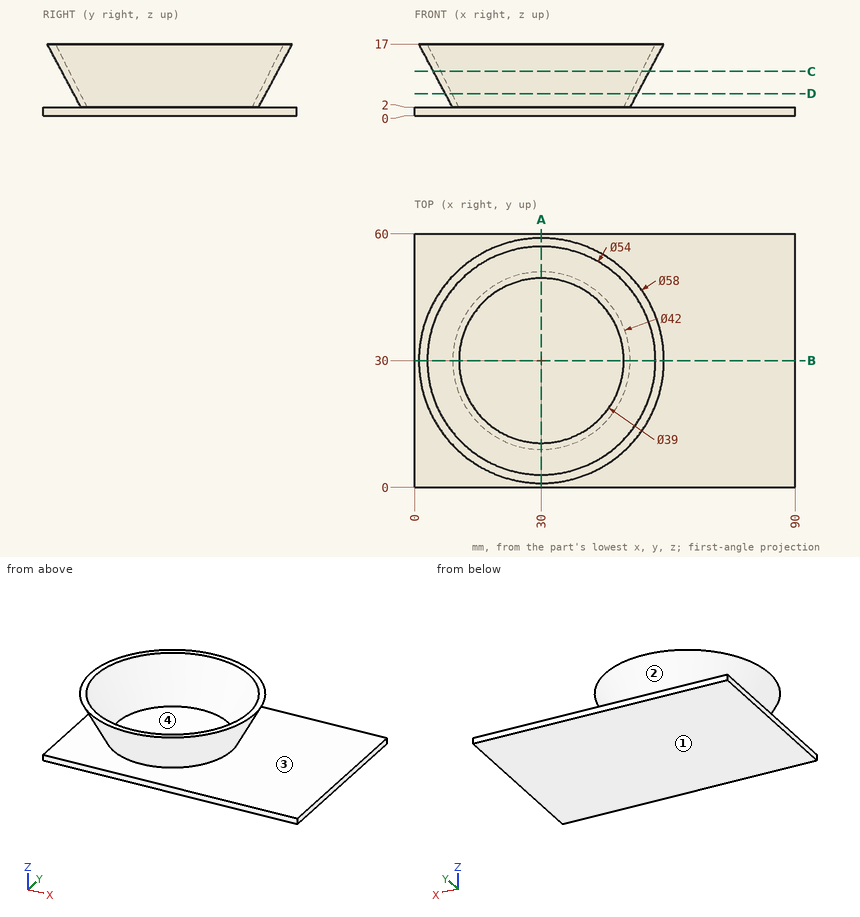
The figure shows three views and two pictorial views of one solid part (mm, origin at its lowest corner). Answer the questions. A direction names the side the tool comes from. Round coordinates to 2 decimals unless told otherwise and drop trailing zeros. Write each loop counter-clockwise with the first axis right and the second up, starting at its lowest first coordinate (ties: lowest second). Pieces come first, ordered by that corner, then holes. Notation, with made-up numbers: (-36, 64) - (4, 64) arc R25 cw to (4, 85) - close; hole circle Ø10 at (20.25, -7.75). An arc over 180 degrees is marked (long way). Use one line per item in the form item = value. Start each with the question number.
Item 1: Determine the mould class of the marked faces 3 and 4 for opening direction X: +X half, -X half, draft (parallel to the pull), parting line (faces both ways), or undercut.
Item 2: A cutting plane is placed at B-B (y = 30). Write down the section's boundary in (x, z), plus the area to 4 significant figures.
Item 3: A cutting plane is placed at D-D (z = 5.25). Write down the section's boundary in (x, y) (3 decimals), plus the area to 3 significant figures.
Item 4: A cutting plane is placed at A-A (x = 30). Write down the section's boundary in (y, z), plus the area to 4 significant figures.
Item 5: Find the intervals of material crossed by line 1 (X direction, y = 39, z = 14.75); line 2 (X direction, y = 15.5, z = 8.75); line 3 (Y direction, x = 16.5, z = 7.5), in increasing order. Write a range as [from, to].
Item 6: A cutting plane is placed at C-C (z = 10.5). Write down the section's boundary in (x, y), plus the area to 3 significant figures.
Item 7: A tool of negligible diameter and unlimited length cuts with its end or side. For the marked faces 1 and 2, from which of +Z, -Z, +X, -X, +Y, -Y can it reach the whole face along a straight path? Write none if from no direction.
Item 8: Flat-ended cylindrical pins translate along their axes: pin 1 Ø8 at (x, y) = (32.5, 52.5) entering from +Z; pin 2 Ø6 at (x, z) = (35.5, 9) entering from -Y; pin 3 Ø19.5 at (x, y) = (29, 20.5) entering from +Z. Find the tip coordinate at first contact, or state that the pin passes through.
The answers:
q1.face_3 = draft
q1.face_4 = undercut
q2.outline = (0, 0) - (90, 0) - (90, 2) - (51, 2) - (59, 17) - (57, 17) - (49.5, 2) - (10.5, 2) - (3, 17) - (1, 17) - (9, 2) - (0, 2) - close
q2.area = 232.5 mm^2
q3.outline = circle Ø45.467 at (30, 30); hole circle Ø42.25 at (30, 30)
q3.area = 222 mm^2
q4.outline = (0, 0) - (60, 0) - (60, 2) - (51, 2) - (59, 17) - (57, 17) - (49.5, 2) - (10.5, 2) - (3, 17) - (1, 17) - (9, 2) - (0, 2) - close
q4.area = 172.5 mm^2
q5.line_1 = [3.7, 5.74], [54.26, 56.3]
q5.line_2 = [10.13, 12.31], [47.69, 49.87]
q5.line_3 = [10.24, 12.31], [47.69, 49.76]
q6.outline = circle Ø51.07 at (30, 30); hole circle Ø47.5 at (30, 30)
q6.area = 276 mm^2
q7.face_1 = -Z, +X, -X, +Y, -Y
q7.face_2 = none
q8.pin_1 = 16.28
q8.pin_2 = 4.15
q8.pin_3 = 2
